```python
from build123d import *

# Parameters (mm, degrees)
SKETCH1_R           = 1.5
BOSS_EXTRUDE1_DEPTH = 3.175


with BuildPart() as part:
    # Sketch1 → Boss-Extrude1 (new body)
    with BuildSketch(Plane(origin=(0, 0, 0), x_dir=(1, 0, 0), z_dir=(0, 1, 0))):
        with BuildLine():
            Line((7.858300919, -2.484134681), (13.014762042, -2.484134681))
            ThreePointArc((13.014762042, -2.484134681), (15.743606535, 0.244709812), (13.014762042, 2.973554305))
            Line((13.014762042, 2.973554305), (7.969118099, 2.744709812))
            ThreePointArc((7.969118099, 2.744709812), (5.624188125, 5.376129638), (2.206241257, 6.236772472))
            Line((2.206241257, 6.236772472), (-0.371989304, 10.702398798))
            ThreePointArc((-0.371989304, 10.702398798), (-4.099660205, 11.701225206), (-5.098486612, 7.973554305))
            Line((-5.098486612, 7.973554305), (-2.377479496, 3.718320719))
            ThreePointArc((-2.377479496, 3.718320719), (-3.483890927, 0.371841879), (-2.520256051, -3.018508355))
            Line((-2.520256051, -3.018508355), (-5.098486612, -7.484134681))
            ThreePointArc((-5.098486612, -7.484134681), (-4.099660205, -11.211805582), (-0.371989304, -10.212979174))
            Line((-0.371989304, -10.212979174), (1.952647522, -5.728901095))
            ThreePointArc((1.952647522, -5.728901095), (5.403988927, -5.013842081), (7.858300919, -2.484134681))
        make_face()
        Polygon((3.958137715, 2.744709812), (5.401513388, 0.244709812), (3.958137715, -2.255290188), (1.071386369, -2.255290188), (-0.371989304, 0.244709812), (1.071386369, 2.744709812), align=None, mode=Mode.SUBTRACT)
        with Locations(Location((13.014762042, 0.244709812, 0), (0, 0, 270))):
            Circle(SKETCH1_R, mode=Mode.SUBTRACT)
        with Locations(Location((-2.735237958, 9.337976552, 0), (0, 0, 270))):
            Circle(SKETCH1_R, mode=Mode.SUBTRACT)
        with Locations(Location((-2.735237958, -8.848556928, 0), (0, 0, 270))):
            Circle(SKETCH1_R, mode=Mode.SUBTRACT)
    extrude(amount=BOSS_EXTRUDE1_DEPTH)


solid = part.part
```
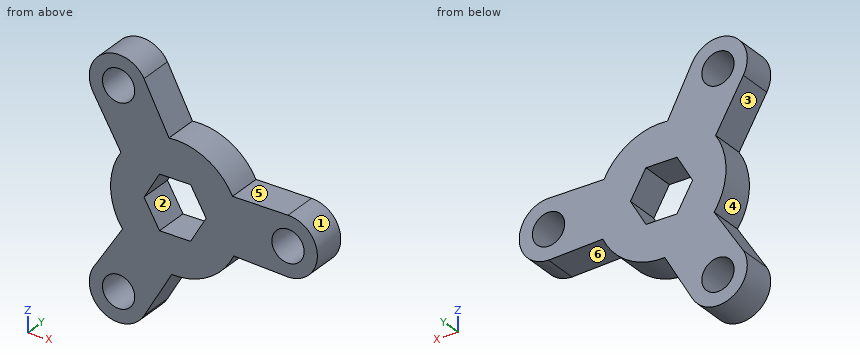
Input: part model. Units: mm. Frame: model coordinates. Face numbers are marked on the shaded views. A direction names the side the tool comes from. Round coordinates to 2 decimals unless told otherwise and drop trailing zeros. Loops run counter-clockwise (first coordinate to the right, second up) from the corner with the lowest first, then second, coordinate; pieces in that order, holes last. Notation, with made-up numbers: (-13, 64.25) -> (24, 64.25) arc R21 cw to (24, 84.25) -> close; hole circle Ø4 at (-16.75, 84.25). An arc over 180 degrees is marked (long way). Write each question's results on one line, items separated by ' | '.
1. Section C-C (z = 9.5). Return loops of the section in (x, y) (3 decimals), and give its area (3 significant figures).
Geometry results:
outline: (-5.385, 0) -> (-4.086, 0) -> (-4.086, 3.175) -> (-5.385, 3.175) -> close; (-1.384, 0) -> (-0.002, 0) -> (-0.002, 3.175) -> (-1.384, 3.175) -> close | area: 8.51 mm2
2. Section B-B (z = 0.75). Return loops of the section in (x, y) (1 decimal), and give its area (3 significant figures).
Geometry results:
outline: (-3.4, 0) -> (0.2, 0) -> (0.2, 3.2) -> (-3.4, 3.2) -> close; (4.8, 0) -> (11.9, 0) -> (11.9, 3.2) -> (4.8, 3.2) -> close; (14.1, 0) -> (15.6, 0) -> (15.6, 3.2) -> (14.1, 3.2) -> close | area: 38.4 mm2
3. Mould query, pull axis Z, two halves, no side actions, for the marked faces 3, 4, 5 and 6. Classes: +Z half, -Z half, draft (parallel to the pull), parting line (faces both ways), or undercut.
Geometry results:
face 3: undercut | face 4: undercut | face 5: +Z half | face 6: -Z half
4. Ray query, line 1 (X direction, y = 2, z = -1.25); line 2 (X direction, y = 0.15, z = 2); line 3 (Z direction, x = 1.5, y = 0.85). Return the intervals inside material, ascending. Write a range as from..to.
Geometry results:
line 1: -3.4..0.21, 4.82..11.9, 14.13..15.55 | line 2: -3.05..0.92, 4.11..14.57 | line 3: -7.46..-2.74, 2.26..6.6
5. Section A-A (x = 4.75). Return loops of the section in (y, z) (3 decimals), and give its area (3 significant figures).
Geometry results:
outline: (0, -5.813) -> (3.175, -5.813) -> (3.175, -1.373) -> (0, -1.373) -> close; (0, 0.884) -> (3.175, 0.884) -> (3.175, 5.323) -> (0, 5.323) -> close | area: 28.2 mm2
6. Section D-D (y = 1.1). Return loops of the section in (x, z), and give its area (3 significant figures).
Geometry results:
outline: (-5.1, -7.97) arc R2.73 ccw to (-0.37, -10.7) -> (2.21, -6.24) arc R6 ccw to (7.97, -2.74) -> (13.01, -2.97) arc R2.73 ccw to (13.01, 2.48) -> (7.86, 2.48) arc R6 ccw to (1.95, 5.73) -> (-0.37, 10.21) arc R2.73 ccw to (-5.1, 7.48) -> (-2.52, 3.02) arc R6 ccw to (-2.38, -3.72) -> close; hole circle Ø3 at (-2.74, -9.34); hole circle Ø3 at (-2.74, 8.85); hole (-0.37, -0.24) -> (1.07, -2.74) -> (3.96, -2.74) -> (5.4, -0.24) -> (3.96, 2.26) -> (1.07, 2.26) -> close; hole circle Ø3 at (13.01, -0.24) | area: 181 mm2
7. First-contact query: P1, Ø3.5, axis at x = 13.01, z = -0.24, coming from the +Y side (3 decimals); P2, Ø0.9, axis at x = 2.5, y = 1, coming from the +Z side. Flat tips, straight axial feed; report the tip coordinate or a pass-through.
Geometry results:
P1: y = 3.175 | P2: z = 5.76
8. Set-up query: the marked faces 1 and 2. Return all of +Z, -Z, +X, -X, +Y, -Y with unobstructed straight access to the full face (end or side cutting, diameter ignored); none if empty.
Geometry results:
face 1: +X, +Y, -Y | face 2: +Y, -Y
